Verification items for the finished model (mm, model axes). Face numbers are marked on the shaded views. A direction names the side the tool comes from. Give positions to 0.01 mm unless a question says otherwise; leave off trailing zeros. Write each loop counter-clockwise with the first axis right and the second up, starting at its lowest first coordinate (ties: lowest second). Pieces come first, ordered by that corner, then holes. Notation, with made-up numbers: (61, 88.25) -> (93, 88.25) arc R18 ccw to (93, 117.25) -> close; hole circle Ø4 at (89.5, 7). An arc over 180 degrees is marked (long way). Answer as CSV lines item,"result".
```python
from build123d import *

# Parameters (mm, degrees)
SKETCH1_R            = 27.5
BOSS_EXTRUDE1_DEPTH  = 15
BOSS_EXTRUDE3_DEPTH  = 2.5
FILLET2_R            = 1.5
SKETCH4_R            = 3
CUT_EXTRUDE1_DEPTH   = 5
SKETCH5_R            = 15
CUT_EXTRUDE2_DEPTH   = 15
BOSS_EXTRUDE6_DEPTH  = 2.5
SKETCH8_R            = 2
CUT_EXTRUDE3_DEPTH   = 17.5
SKETCH9_R            = 3.5
SKETCH9_R_2          = 2
CUT_EXTRUDE4_DEPTH   = 4
SKETCH10_R           = 2
CUT_EXTRUDE5_DEPTH   = 2.5
BOSS_EXTRUDE14_START = -5.5
SKETCH14_R           = 30
BOSS_EXTRUDE14_DEPTH = 5.5


with BuildPart() as part:
    # Sketch1 → Boss-Extrude1 (new body)
    with BuildSketch(Plane(origin=(0, 0, 0), x_dir=(1, 0, 0), z_dir=(0, 1, 0))):
        with Locations(Location((0, 0, 0), (0, 0, 270))):
            Circle(SKETCH1_R)
    extrude(amount=BOSS_EXTRUDE1_DEPTH)

    # Sketch3 → Boss-Extrude3 (add)
    with BuildSketch(Plane(origin=(0, 15, 0), x_dir=(1, 0, 0), z_dir=(0, 1, 0))):
        with BuildLine():
            ThreePointArc((0, -24.315632832), (-21.5, 0), (0, 24.315632832))
            Line((0, 24.315632832), (0, 27.5))
            ThreePointArc((0, 27.5), (-27.5, 0), (0, -27.5))
            Line((0, -27.5), (0, -24.315632832))
        make_face()
    extrude(amount=BOSS_EXTRUDE3_DEPTH)

    # Fillet2
    # the kernel refuses this fillet: 1.5 mm, written as the material it takes off along each edge
    with BuildSketch(Plane(origin=(0, 15, 24.315632832), x_dir=(0, 0, 1), z_dir=(0, 1, 0))) as fillet2_piece_1:
        with BuildLine():
            CenterArc((1.291983223, -1.5), FILLET2_R, 90, 80.0332337)
            ThreePointArc((-0.185379242, -1.240384615), (-0.084751372, -0.621378703), (0, 0))
            Line((0, 0), (1.291983223, 0))
        make_face()
    extrude(amount=5.729958058, mode=Mode.SUBTRACT)
    with BuildSketch(Plane(origin=(0, 15, -24.315632832), x_dir=(0, 0, -1), z_dir=(0, 1, 0))) as fillet2_piece_2:
        with BuildLine():
            CenterArc((1.291983223, 1.5), FILLET2_R, 189.9667663, 80.0332337)
            ThreePointArc((-0.185379242, 1.240384615), (-0.084751372, 0.621378703), (0, 0))
            Line((0, 0), (1.291983223, 0))
        make_face()
    extrude(amount=5.729958058, mode=Mode.SUBTRACT)
    with BuildSketch(Plane(origin=(0, 15, -27.5), x_dir=(-0.9995835162017269, 0, 0.02885817280757429), z_dir=(0, 1, 0))) as fillet2_piece_3:
        with BuildLine():
            CenterArc((1.543912245, 1.499375274), FILLET2_R, 178.34631891, 93.30736218)
            Line((0.044536971, 1.542662534), (0, 0))
            ThreePointArc((0, 0), (0.793599752, -0.011453304), (1.587199504, 0))
        make_face()
    extrude(amount=6.467998761, mode=Mode.SUBTRACT)
    with BuildSketch(Plane(origin=(0, 15, 27.5), x_dir=(-0.999583516201727, 0, -0.028858172807574353), z_dir=(0, 1, 0))) as fillet2_piece_4:
        with BuildLine():
            CenterArc((1.543912245, -1.499375274), FILLET2_R, 88.34631891, 93.30736218)
            Line((0.044536971, -1.542662534), (0, 0))
            ThreePointArc((0, 0), (0.793599752, 0.011453304), (1.587199504, 0))
        make_face()
    extrude(amount=6.467998761, mode=Mode.SUBTRACT)

    # Sketch4 → Cut-Extrude1 (cut)
    with BuildSketch(Plane(origin=(0, 15, 0), x_dir=(1, 0, 0), z_dir=(0, 1, 0))):
        with Locations(Location((-16.75, 0, 0), (0, 0, 270))):
            Circle(SKETCH4_R)
        with Locations(Location((12.875, 17.104001725, 0), (0, 0, 270))):
            Circle(SKETCH4_R)
        with Locations(Location((12.875, -17.104001725, 0), (0, 0, 270))):
            Circle(SKETCH4_R)
    extrude(amount=-CUT_EXTRUDE1_DEPTH, mode=Mode.SUBTRACT)

    # Sketch5 → Cut-Extrude2 (cut)
    with BuildSketch(Plane(origin=(0, 15, 0), x_dir=(1, 0, 0), z_dir=(0, 1, 0))):
        with Locations(Location((3, 0, 0), (0, 0, 270))):
            Circle(SKETCH5_R)
    extrude(amount=-CUT_EXTRUDE2_DEPTH, mode=Mode.SUBTRACT)

    # Sketch7 → Boss-Extrude6 (add)
    with BuildSketch(Plane.XZ):
        with BuildLine():
            ThreePointArc((0, 24.315632832), (-21.5, 0), (0, -24.315632832))
            Line((0, -24.315632832), (0, -14.696938457))
            ThreePointArc((0, -14.696938457), (-12, 0), (0, 14.696938457))
            Line((0, 14.696938457), (0, 24.315632832))
        make_face()
        with BuildLine():
            Line((0, -14.696938457), (0, -24.315632832))
            ThreePointArc((0, -24.315632832), (19.228832367, -18.354154843), (27.5, 0))
            ThreePointArc((27.5, 0), (19.228832367, 18.354154843), (0, 24.315632832))
            Line((0, 24.315632832), (0, 14.696938457))
            ThreePointArc((0, 14.696938457), (12.486832981, 11.618950039), (18, 0))
            ThreePointArc((18, 0), (12.486832981, -11.618950039), (0, -14.696938457))
        make_face()
    extrude(amount=BOSS_EXTRUDE6_DEPTH)

    # Sketch8 → Cut-Extrude3 (cut)
    with BuildSketch(Plane(origin=(0, 15, 0), x_dir=(1, 0, 0), z_dir=(0, 1, 0))):
        with Locations(Location((-6.875, 17.104001725, 0), (0, 0, 270))):
            Circle(SKETCH8_R)
        with Locations(Location((-6.875, -17.104001725, 0), (0, 0, 270))):
            Circle(SKETCH8_R)
        with Locations(Location((22.75, 0, 0), (0, 0, 270))):
            Circle(SKETCH8_R)
    extrude(amount=-CUT_EXTRUDE3_DEPTH, mode=Mode.SUBTRACT)

    # Sketch9 → Cut-Extrude4 (cut)
    # profile 1 of 3: a face of its own
    with BuildSketch(Plane(origin=(0, 15, 0), x_dir=(1, 0, 0), z_dir=(0, 1, 0))):
        with Locations(Location((-6.875, 17.104001725, 0), (0, 0, 270))):
            Circle(SKETCH9_R)
        with Locations(Location((-6.875, 17.104001725, 0), (0, 0, 270))):
            Circle(SKETCH9_R_2, mode=Mode.SUBTRACT)
    # profile 2 of 3: a face of its own
    with BuildSketch(Plane(origin=(0, 15, 0), x_dir=(1, 0, 0), z_dir=(0, 1, 0))):
        with Locations(Location((22.75, 0, 0), (0, 0, 270))):
            Circle(SKETCH9_R)
        with Locations(Location((22.75, 0, 0), (0, 0, 270))):
            Circle(SKETCH9_R_2, mode=Mode.SUBTRACT)
    # profile 3 of 3: a face of its own
    with BuildSketch(Plane(origin=(0, 15, 0), x_dir=(1, 0, 0), z_dir=(0, 1, 0))):
        with Locations(Location((-6.875, -17.104001725, 0), (0, 0, 270))):
            Circle(SKETCH9_R)
        with Locations(Location((-6.875, -17.104001725, 0), (0, 0, 270))):
            Circle(SKETCH9_R_2, mode=Mode.SUBTRACT)
    extrude(amount=-CUT_EXTRUDE4_DEPTH, mode=Mode.SUBTRACT)

    # Sketch10 → Cut-Extrude5 (cut)
    with BuildSketch(Plane(origin=(0, 10, 0), x_dir=(1, 0, 0), z_dir=(0, 1, 0))):
        with Locations(Location((-16.75, 0, 0), (0, 0, 270))):
            Circle(SKETCH10_R)
        with Locations(Location((12.875, 17.104001725, 0), (0, 0, 270))):
            Circle(SKETCH10_R)
        with Locations(Location((12.875, -17.104001725, 0), (0, 0, 270))):
            Circle(SKETCH10_R)
    extrude(amount=-CUT_EXTRUDE5_DEPTH, mode=Mode.SUBTRACT)

    # Sketch14 → Boss-Extrude14 (add)
    # profile 1 of 4: a face of its own
    with BuildSketch(Plane(origin=(0, 17.5, 0), x_dir=(1, 0, 0), z_dir=(0, 1, 0)).offset(BOSS_EXTRUDE14_START)):
        with Locations(Location((0, 0, 0), (0, 0, 270))):
            Circle(SKETCH14_R)
        with BuildLine():
            ThreePointArc((-1.586538462, 27.454196322), (18.876178007, 19.99849754), (27.5, 0))
            ThreePointArc((27.5, 0), (18.876178007, -19.99849754), (-1.586538462, -27.454196322))
            ThreePointArc((-1.586538462, -27.454196322), (-27.5, 0), (-1.586538462, 27.454196322))
        make_face(mode=Mode.SUBTRACT)
    # profile 2 of 4: a face of its own
    with BuildSketch(Plane(origin=(0, 17.5, 0), x_dir=(1, 0, 0), z_dir=(0, 1, 0)).offset(BOSS_EXTRUDE14_START)):
        with BuildLine():
            ThreePointArc((-1.240384615, 24.13025359), (-0.351213014, 24.64310143), (0, 25.607616055))
            Line((0, 25.607616055), (0, 25.956694705))
            ThreePointArc((0, 25.956694705), (-0.470390291, 27.047521843), (-1.586538462, 27.454196322))
            ThreePointArc((-1.586538462, 27.454196322), (-27.5, 0), (-1.586538462, -27.454196322))
            ThreePointArc((-1.586538462, -27.454196322), (-0.470390291, -27.047521843), (0, -25.956694705))
            Line((0, -25.956694705), (0, -25.607616055))
            ThreePointArc((0, -25.607616055), (-0.351213014, -24.64310143), (-1.240384615, -24.13025359))
            ThreePointArc((-1.240384615, -24.13025359), (-21.5, 0), (-1.240384615, 24.13025359))
        make_face()
    # profile 3 of 4: a face of its own
    with BuildSketch(Plane(origin=(0, 17.5, 0), x_dir=(1, 0, 0), z_dir=(0, 1, 0)).offset(BOSS_EXTRUDE14_START)):
        with BuildLine():
            ThreePointArc((-1.240384615, 24.13025359), (18.753738872, 18.763520766), (27.5, 0))
            ThreePointArc((27.5, 0), (18.876178007, 19.99849754), (-1.586538462, 27.454196322))
            ThreePointArc((-1.586538462, 27.454196322), (-0.470390291, 27.047521843), (0, 25.956694705))
            Line((0, 25.956694705), (0, 25.607616055))
            ThreePointArc((0, 25.607616055), (-0.351213014, 24.64310143), (-1.240384615, 24.13025359))
        make_face()
    # profile 4 of 4: a face of its own
    with BuildSketch(Plane(origin=(0, 17.5, 0), x_dir=(1, 0, 0), z_dir=(0, 1, 0)).offset(BOSS_EXTRUDE14_START)):
        with BuildLine():
            ThreePointArc((-1.586538462, -27.454196322), (18.876178007, -19.99849754), (27.5, 0))
            ThreePointArc((27.5, 0), (18.753738872, -18.763520766), (-1.240384615, -24.13025359))
            ThreePointArc((-1.240384615, -24.13025359), (-0.351213014, -24.64310143), (0, -25.607616055))
            Line((0, -25.607616055), (0, -25.956694705))
            ThreePointArc((0, -25.956694705), (-0.470390291, -27.047521843), (-1.586538462, -27.454196322))
        make_face()
    extrude(amount=BOSS_EXTRUDE14_DEPTH)


solid = part.part
```
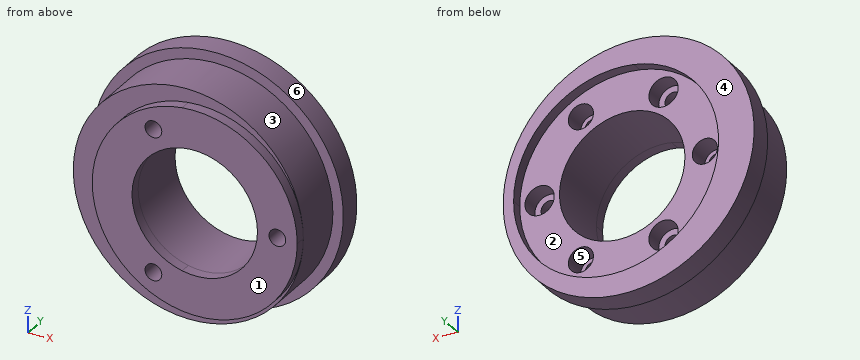
1) Section check D-D (y = 6). Record the boundary of the cut face in (x, z) (3 decimals), and give its area (3 significant figures).
Reported:
outline,"circle Ø55 at (0, 0); hole circle Ø30 at (3, 0); hole circle Ø4 at (-6.875, -17.104); hole circle Ø4 at (-6.875, 17.104); hole circle Ø4 at (22.75, 0)"
area,"1,630 mm²"
2) Depth check by flat-ended pin: pin 1 (12 mm diameter, centred on y = 1.5, z = -5, fed in from +X); pin 2 (4 mm diameter, centred on x = -22.5, y = 5, fed in from +Z); pin 3 (5 mm diameter, centred on y = 5, z = -16.5, fed in from +X). Enter the tip coordinate at first touch or a pass-through.
Reported:
pin 1,"x = 27.5"
pin 2,"z = 18.33"
pin 3,"x = 23.67"
3) Draft check along X on the marked faces 4, 5 and 6. Enter one of: +X half, -X half, draft (parallel to the pull), parting line (faces both ways), or undercut.
Reported:
face 4,"draft"
face 5,"undercut"
face 6,"parting line"
4) Section check C-C (y = 16.25). Record the boundary of the cut face in (x, z), and give its area (3 significant figures).
Reported:
outline,"circle Ø60 at (0, 0); hole circle Ø49 at (3, 0)"
area,"942 mm²"
5) Scan lines: line 1 along X through (y, z) = (5.5, 0); line 2 along X through (y, z) = (14, 18.5); line 3 along X through (y, z) = (-1.25, -10.5). Record each from-to range of solid material in increasing order.
Reported:
line 1,"-27.5 to -12, 18 to 20.75, 24.75 to 27.5"
line 2,"-23.62 to -10.08, -3.67 to 10.22, 15.53 to 23.62"
line 3,"-19.14 to -7.71, 13.71 to 25.14"
6) Section check A-A (x = 22.75). Record the boundary of the cut face in (y, z), and give its area (3 significant figures).
Reported:
outline,"(-2.5, -14.5) -> (0, -14.5) -> (0, -15.45) -> (12, -15.45) -> (12, -19.56) -> (17.5, -19.56) -> (17.5, -14.5) -> (15, -14.5) -> (15, -3.5) -> (11, -3.5) -> (11, -2) -> (-2.5, -2) -> close; (-2.5, 2) -> (11, 2) -> (11, 3.5) -> (15, 3.5) -> (15, 14.5) -> (17.5, 14.5) -> (17.5, 19.56) -> (12, 19.56) -> (12, 15.45) -> (0, 15.45) -> (0, 14.5) -> (-2.5, 14.5) -> close"
area,"504 mm²"
7) Section check B-B (z = -12). Record the boundary of the cut face in (x, y), and give its area (3 significant figures).
Reported:
outline,"(-27.5, 12) -> (-24.74, 12) -> (-24.74, 0) -> (-18.36, 0) -> (-18.36, -2.5) -> (-6, -2.5) -> (-6, 15) -> (-18.36, 15) -> (-18.36, 17.5) -> (-27.5, 17.5) -> close; (12, -2.5) -> (24.36, -2.5) -> (24.36, 0) -> (24.74, 0) -> (24.74, 12) -> (27.5, 12) -> (27.5, 17.5) -> (24.36, 17.5) -> (24.36, 15) -> (12, 15) -> close"
area,"581 mm²"
8) Tool access check on the marked faces 1, 2 and 3. Record the directions out of +Z, -Z, +X, -X, +Y, -Y that give a thin tool (end or side, any length) a straight path to the whole face; none if there is none.
Reported:
face 1,"+Z, -Z, +X, -X, -Y"
face 2,"+Y"
face 3,"-Y"
